Can you work these out from the model? Positions are in its coordinate system, mm. Face numbers are marked on the shaded views. A direction names the side the tool comes from. Give positions to 0.01 mm unless a question says otherwise; leave off trailing zeros. Loops run counter-clockwise (first coordinate to the right, second up) from the corner with the lowest first, then second, coordinate; pieces in that order, holes last. Notation, with made-up numbers: (46.25, 39) -> (89.25, 39) arc R24 cw to (89.25, 65) -> close; hole circle Ø11 at (19, 37.25). An arc over 180 degrees is marked (long way). Return JSON: item names as keys, results as strings. Group by question number.
Q1. Suppose I cut it at C-C, the plane x = 0. Please give me the cut outline in (y, z), and give its area (3 significant figures).
Q2. I need wall thicknesses on line 1 along Y through (x, z) = (-50.8, 21.5); line 2 along X through (y, z) = (50.8, 29); line 3 along Z through (x, y) = (-8.5, 58). Which ranges of each line are inside material? Lowest first, please. Write a range as [from, to].
Q3. Suppose I cut it at B-B, the plane y = 0. Please give me the cut outline in (x, z).
Q4. Suppose I cut it at A-A, the plane z = 21.5. Please give me the cut outline in (x, y).
Q5. Which directions (+Z, -Z, +X, -X, +Y, -Y) give clear straight access to the entire face, cutting with the end or side of a thin tool? Please do the marked faces 1 and 2.
```python
from build123d import *

# Parameters (mm, degrees)
F1_W     = 127
F1_H     = 38.1
F2_DEPTH = 63.5
F5_DEPTH = 50.8
F7_DEPTH = 50.8


with BuildPart() as f2:
    # F1 (on Front) → F2 (new body, symmetric)
    with BuildSketch(Plane.XZ):
        with Locations((-0.005746, 19.05)):
            Rectangle(F1_W, F1_H)
    extrude(amount=F2_DEPTH, both=True)

    # F0 (on Front) → F3 (revolve, cut)
    with BuildSketch(Plane.XZ):
        Polygon((53.190532, 10.998523), (38.1, 2.286), (0, 2.286), (0, 0), (132.006165, 0), (132.006165, 10.998523), align=None)
    revolve(axis=Axis((0, 0, 1.143), (0, 0, -1)), mode=Mode.SUBTRACT)

    # F4 (on Top) → F5 (cut, symmetric)
    with BuildSketch(Plane.XY):
        with BuildLine():
            Line((-50.8, 44.45), (-50.8, 50.8))
            Line((-50.8, 50.8), (-44.45, 50.8))
            ThreePointArc((-44.45, 50.8), (-55.290128, 55.290128), (-50.8, 44.45))
        make_face()
        with BuildLine():
            Line((-44.45, 50.8), (-50.8, 50.8))
            Line((-50.8, 50.8), (-50.8, 44.45))
            ThreePointArc((-50.8, 44.45), (-46.309872, 46.309872), (-44.45, 50.8))
        make_face()
    extrude(amount=F5_DEPTH, both=True, mode=Mode.SUBTRACT)

    # F6 (on Top) → F7 (cut, symmetric)
    with BuildSketch(Plane.XY):
        with BuildLine():
            ThreePointArc((50.8, -44.45), (46.309872, -46.309872), (44.45, -50.8))
            Line((44.45, -50.8), (50.8, -50.8))
            Line((50.8, -50.8), (50.8, -44.45))
        make_face()
        with BuildLine():
            Line((50.8, -50.8), (44.45, -50.8))
            ThreePointArc((44.45, -50.8), (50.8, -57.15), (57.15, -50.8))
            ThreePointArc((57.15, -50.8), (55.290128, -46.309872), (50.8, -44.45))
            Line((50.8, -44.45), (50.8, -50.8))
        make_face()
    extrude(amount=F7_DEPTH, both=True, mode=Mode.SUBTRACT)


solid = f2.part
```
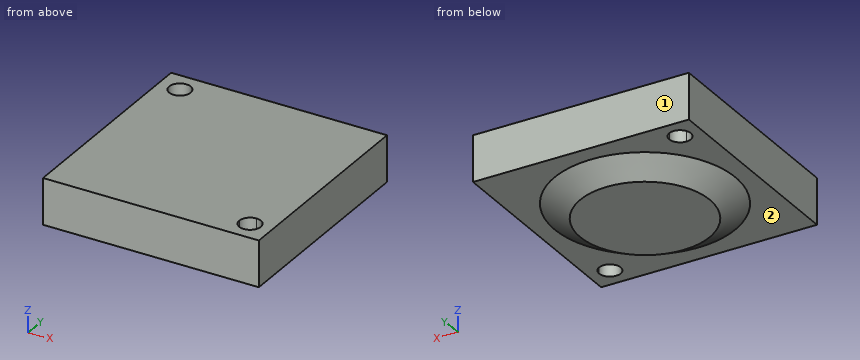
Ans:
{
 "1": {"outline": "(-63.5, 11) -> (-53.19, 11) -> (-38.1, 2.29) -> (38.1, 2.29) -> (53.19, 11) -> (63.5, 11) -> (63.5, 38.1) -> (-63.5, 38.1) -> close", "area": "4,240 mm^2"},
 "2": {"line 1": "y = [-63.5, 44.45], [57.15, 63.5]", "line 2": "x = [-63.51, -57.15], [-44.45, 63.49]", "line 3": "z = [11, 38.1]"},
 "3": {"outline": "(-63.51, 11) -> (-53.19, 11) -> (-38.1, 2.29) -> (38.1, 2.29) -> (53.19, 11) -> (63.49, 11) -> (63.49, 38.1) -> (-63.51, 38.1) -> close"},
 "4": {"outline": "(-63.51, -63.5) -> (63.49, -63.5) -> (63.49, 63.5) -> (-63.51, 63.5) -> close; hole circle Ø12.7 at (-50.8, 50.8); hole circle Ø12.7 at (50.8, -50.8)"},
 "5": {"face 1": "+Z, -Z, +X, -X, +Y", "face 2": "-Z"}
}
